Geometry: see drawing. Coordinates: mm, zero at the bounding-box minimum. Round coordinates to 2 decimals unless told otherwise and drop trailing zeros. Loops run counter-clockwise (first coordinate to the right, second up) from the corner with the lowest first, then second, coordinate; pieces in that order, holes last. Notation, with made-up numbers: M 60.25,81.25 L 91.25,81.25 A17 cw 91.25,101.25 Z; hole C -3,8.5 d6. An arc over 180 degrees is marked long. Answer as a JSON object with one key per item and string values.
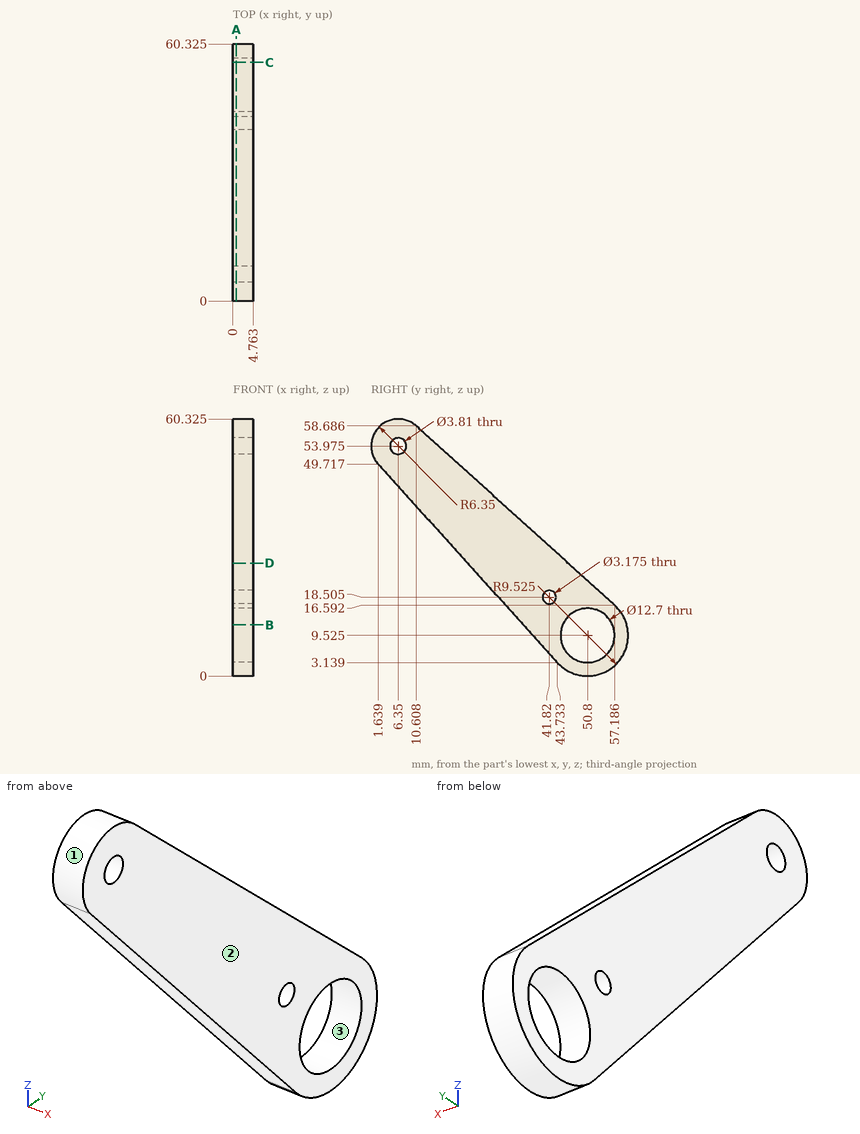
1) Section query A-A (x = 0.85). Count the separate pieces of the cut face and the enclosed holes in it, and give its area (3 significant figures).
Results:
{"separate pieces": "1", "enclosed holes": "3", "area": "1,060 mm2"}
2) Section query D-D (z = 26.5). Return the cut outline in (x, y).
Results:
{"outline": "M 0,22.62 L 4.76,22.62 L 4.76,46.22 L 0,46.22 Z"}
3) Pull-direction query (Y, two-part tool) for the marked faces 1, 2 and 3; classes: +Y half, -Y half, draft (parallel to the pull), parting line (faces both ways), or undercut.
Results:
{"face 1": "parting line", "face 2": "draft", "face 3": "undercut"}
4) Section query B-B (z = 12). Return the cut outline in (x, y) (1 decimal), and give its area (3 significant figures).
Results:
{"outline": "M 0,35.7 L 4.8,35.7 L 4.8,45 L 0,45 Z; M 0,56.6 L 4.8,56.6 L 4.8,60 L 0,60 Z", "area": "59.9 mm2"}
5) Section query C-C (y = 56). Return the cut outline in (x, z) (1 decimal).
Results:
{"outline": "M 0,1.5 L 4.8,1.5 L 4.8,5.9 L 0,5.9 Z; M 0,13.2 L 4.8,13.2 L 4.8,17.7 L 0,17.7 Z"}
6) Pin query (flat end, axial travel): P1, Ø1, axis at x = 3, y = 49.5, coming from the -Z side; P2, Ø2, axis at x = 2.5, y = 38, coming from the +Z side (1 decimal); P3, Ø2, axis at x = 3, y = 47.5, coming from the +Z side; P4, Ø11.5, axis at y = 50.8, z = 9.53, coming from the -X side. Return the tip coordinate at first contact, or that it passes through.
Results:
{"P1": "z = 0.03", "P2": "z = 34.8", "P3": "z = 26.25", "P4": "through"}
7) Ray query, line 1 (Z direction, x = 3.55, y = 45) (1 decimal); line 2 (Z direction, x = 1.9, y = 48) (1 decimal); line 3 (Y direction, x = 0.4, z = 52) (1 decimal). Return the intervals inside material, ascending.
Results:
{"line 1": "2 to 6.9, 12.1 to 27.6", "line 2": "0.4 to 3.8, 15.2 to 24.9", "line 3": "0.3 to 18"}
